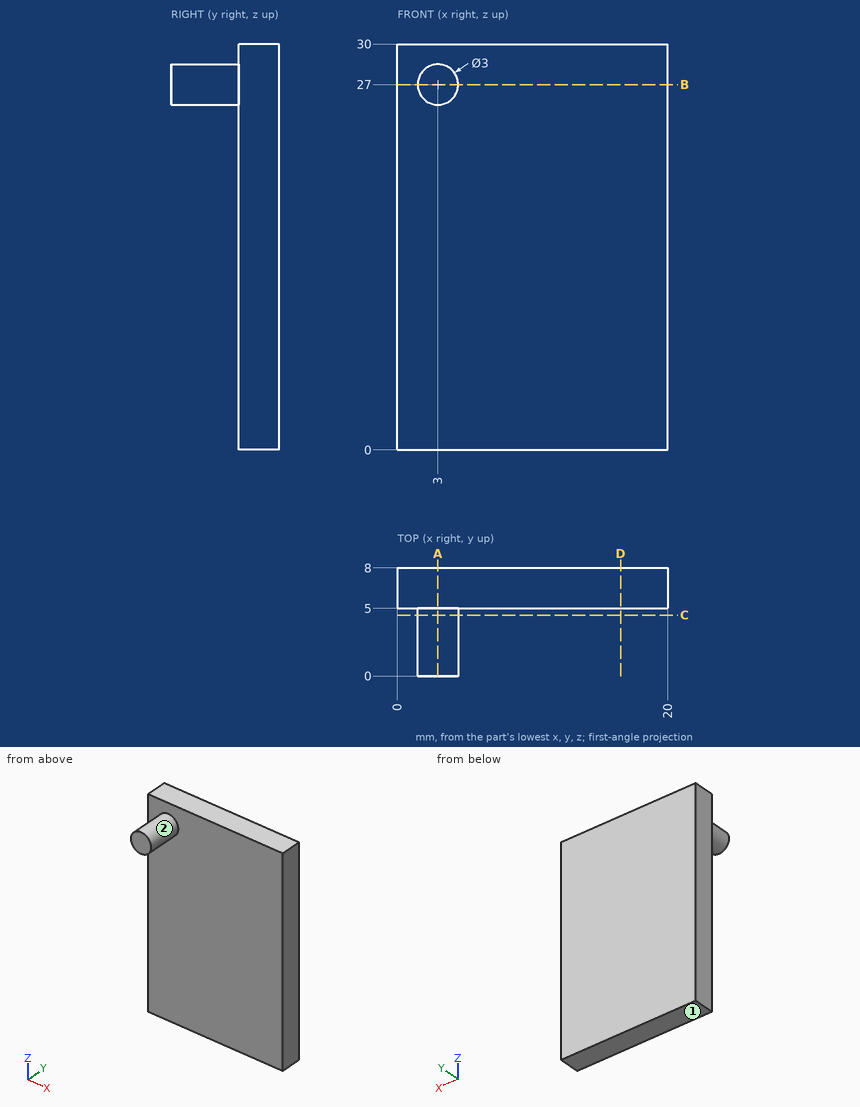
Print and shaded views of the part. All mm, measured from the part's lowest x, y and z. A direction names the side the tool comes from. Coordinates: 2 decimals unless noted, no trailing zeros. Order: outer loops, then holes, each group sorted by start corner. A loop starts at its lowest first (then second) coordinate and runs counter-clockwise, first axis right, second up.
(1) Tool access for the marked faces 1 and 2: list every direction of +Z, -Z, +X, -X, +Y, -Y with a clear straight run to the whole face (end or side of a thin tool).
Check sheet entries:
face 1: -Z, +X, -X, +Y, -Y
face 2: -Y
(2) Slice it at A-A, the plane x = 3. Write the cut outline in (y, z).
Check sheet entries:
outline: (0, 25.5) - (5, 25.5) - (5, 0) - (8, 0) - (8, 30) - (5, 30) - (5, 28.5) - (0, 28.5) - close
(3) Slice it at D-D, the plane x = 16.5. Write the cut outline in (y, z).
Check sheet entries:
outline: (5, 0) - (8, 0) - (8, 30) - (5, 30) - close
(4) Probe L1, parallel to Y at x = 19, z = 14.5; L2, parallel to Z at x = 3, y = 1.5; L3, parallel to Z at x = 2.5, y = 3. List the from-to ranges inside material, lowest first.
Check sheet entries:
L1: y = 5 to 8
L2: z = 25.5 to 28.5
L3: z = 25.59 to 28.41
(5) Pin check, flat tips, straight feed: pin 1 Ø1.5 at (y, z) = (2, 26) entering from -X; pin 2 Ø10 at (x, z) = (7.5, 21.5) entering from -Y; pin 3 Ø2 at (x, y) = (2.5, 3) entering from +Z. Stop position of each tip, or through.
Check sheet entries:
pin 1: stops at x = 1.52
pin 2: stops at y = 5
pin 3: stops at z = 28.5
(6) Slice it at B-B, the plane z = 27. Write the cut outline in (x, y), and give its area (3 significant figures).
Check sheet entries:
outline: (0, 5) - (1.5, 5) - (1.5, 0) - (4.5, 0) - (4.5, 5) - (20, 5) - (20, 8) - (0, 8) - close
area: 75.0 mm2
(7) Slice it at C-C, the plane y = 4.5. Write the cut outline in (x, z).
Check sheet entries:
outline: circle Ø3 at (3, 27)
